Geometry: see drawing. Coordinates: mm, zero at the bounding-box minimum. Coordinates: 2 decimals unless noted, no trailing zeros. Loops run counter-clockwise (first coordinate to the right, second up) from the corner with the lowest first, then second, coordinate; pieces in that order, holes last. Notation, with made-up numbers: (21, 4.5) -> (76, 4.5) arc R10 cw to (76, 21.5) -> close; hole circle Ø9 at (-17, 6.25). An arc over 180 degrees is marked (long way). Answer as a JSON object with one key per item and string values.
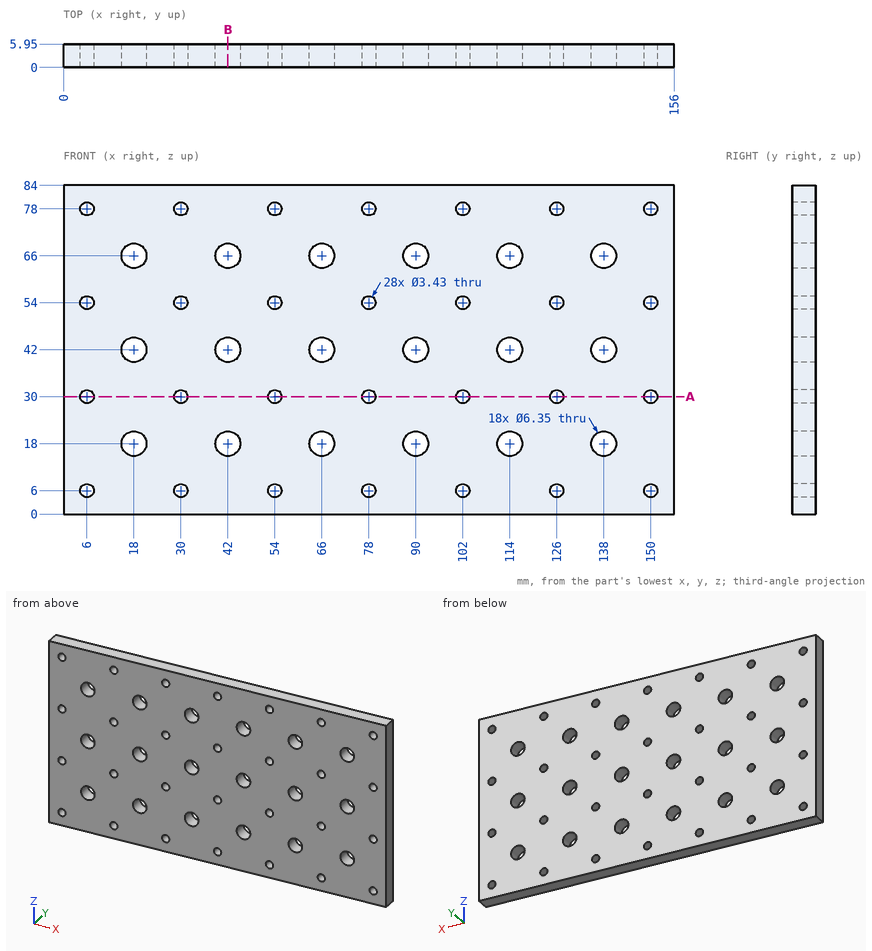
1. Section query A-A (z = 30). Count the separate pieces of the cut face and the enclosed holes in it, plus the area to 3 significant figures.
Reply:
{"separate pieces": "8", "enclosed holes": "0", "area": "785 mm2"}
2. Section query B-B (x = 42). Return loops of the section in (y, z) (3 decimals).
Reply:
{"outline": "(0, 0) -> (5.95, 0) -> (5.95, 14.825) -> (0, 14.825) -> close; (0, 21.175) -> (5.95, 21.175) -> (5.95, 38.825) -> (0, 38.825) -> close; (0, 45.175) -> (5.95, 45.175) -> (5.95, 62.825) -> (0, 62.825) -> close; (0, 69.175) -> (5.95, 69.175) -> (5.95, 84) -> (0, 84) -> close"}
3. Pin query (flat end, axial travel): P1, Ø2, axis at x = 150, z = 30, coming from the -Y side. Return the tip coordinate at first contact, or that it passes through.
Reply:
{"P1": "passes through"}
4. Line query: line 1 along Z through (x, y) = (90, 3.45) (3 decimals); line 2 along Z through (x, y) = (54, 2.4) (3 decimals); line 3 along Z through (x, y) = (149.5, 1.7). Output: solid intervals per line, ascending.
Reply:
{"line 1": "z = 0 to 14.825, 21.175 to 38.825, 45.175 to 62.825, 69.175 to 84", "line 2": "z = 0 to 4.285, 7.715 to 28.285, 31.715 to 52.285, 55.715 to 76.285, 79.715 to 84", "line 3": "z = 0 to 4.36, 7.64 to 28.36, 31.64 to 52.36, 55.64 to 76.36, 79.64 to 84"}
